For this review, take the finished solid that the model builds, in its own axes (mm). Face numbers are marked on the shaded views. A direction names the side the tool comes from. Round coordinates to 2 decimals unless told otherwise and drop trailing zeros. Write each loop counter-clockwise with the first axis right and the second up, starting at its lowest first coordinate (ties: lowest second). Pieces come first, ordered by that corner, then holes.
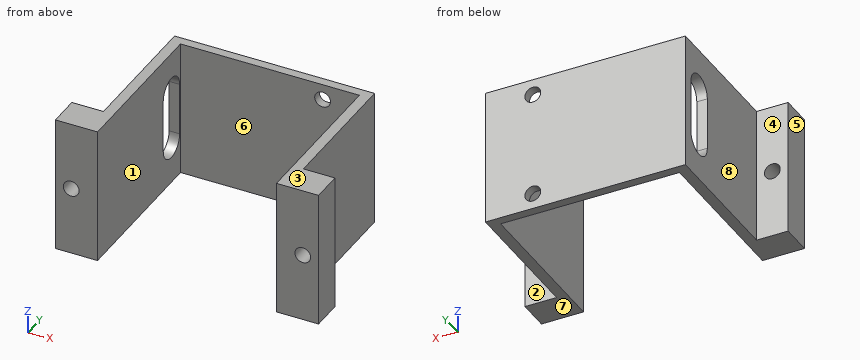
from build123d import *

# Parameters (mm, degrees)
BOSS_EXTRUDE1_DEPTH = 26
SKETCH2_R           = 1.5
CUT_EXTRUDE1_DEPTH  = 48.117375685
SKETCH3_R           = 1.5
CUT_EXTRUDE2_DEPTH  = 45.463468151
CUT_EXTRUDE3_DEPTH  = 10


with BuildPart() as part:
    # Sketch1 → Boss-Extrude1 (new body)
    with BuildSketch(Plane.XY):
        Polygon((-25, -16), (-17, -16), (-17, 14.315789474), (17, 14.315789474), (17, -16), (25, -16), (25, -10), (19, -10), (19, 16), (-19, 16), (-19, -10), (-25, -10), align=None)
    extrude(amount=BOSS_EXTRUDE1_DEPTH)

    # Sketch2 → Cut-Extrude1 (cut, through all)
    with BuildSketch(Plane.XZ.offset(-14.315789474)):
        with Locations(Location((10, 23, 0), (0, 0, 270))):
            Circle(SKETCH2_R)
        with Locations(Location((10, 3, 0), (0, 0, 270))):
            Circle(SKETCH2_R)
    extrude(amount=-CUT_EXTRUDE1_DEPTH, mode=Mode.SUBTRACT)

    # Sketch3 → Cut-Extrude2 (cut, through all)
    with BuildSketch(Plane(origin=(0, -10, 0), x_dir=(1, 0, 0), z_dir=(0, 1, 0))):
        with Locations(Location((22, -13, 0), (0, 0, 180))):
            Circle(SKETCH3_R)
        with Locations(Location((-22, -13, 0), (0, 0, 180))):
            Circle(SKETCH3_R)
    extrude(amount=-CUT_EXTRUDE2_DEPTH, mode=Mode.SUBTRACT)

    # Sketch4 → Cut-Extrude3 (cut)
    with BuildSketch(Plane.ZY.offset(19)):
        with BuildLine():
            Line((8, 14), (18, 14))
            ThreePointArc((18, 14), (21, 11), (18, 8))
            Line((18, 8), (8, 8))
            ThreePointArc((8, 8), (5, 11), (8, 14))
        make_face()
    extrude(amount=-CUT_EXTRUDE3_DEPTH, mode=Mode.SUBTRACT)


solid = part.part
(1) We need section A-A, the plane z = 3. Give the boundary of the cut face in (x, y).
Geometry check:
outline: (-25, -16) - (-17, -16) - (-17, 14.32) - (8.5, 14.32) - (8.5, 16) - (-19, 16) - (-19, -10) - (-25, -10) - close; (11.5, 14.32) - (17, 14.32) - (17, -16) - (25, -16) - (25, -10) - (19, -10) - (19, 16) - (11.5, 16) - close
(2) We need section D-D, the plane z = 13. Give the boundary of the cut face in (x, y).
Geometry check:
outline: (-25, -16) - (-23.5, -16) - (-23.5, -10) - (-25, -10) - close; (-20.5, -16) - (-17, -16) - (-17, 8) - (-19, 8) - (-19, -10) - (-20.5, -10) - close; (-19, 14) - (-17, 14) - (-17, 14.32) - (17, 14.32) - (17, -16) - (20.5, -16) - (20.5, -10) - (19, -10) - (19, 16) - (-19, 16) - close; (23.5, -16) - (25, -16) - (25, -10) - (23.5, -10) - close
(3) Mouldability with a two-part tool opening along X and no side actions: class the marked faces 6, 7 and 8 as pulls with the +X half, pulls with the -X half, needs draft (parallel to the pull), parting line crosses it, or undercut.
Geometry check:
face 6: undercut
face 7: needs draft
face 8: pulls with the -X half
(4) For pin 1 Ø6 at (y, z) = (-9.5, 13) entering from -X; pin 2 Ø3 at (x, z) = (13, 16) entering from -Y; pin 3 Ø5 at (x, z) = (22, 10) entering from +Y; pin 4 Ø1 at (y, z) = (-2.5, 7.5) entering from -X, all flat-tipped, find the tip position at first contact; note any pin that passes through.
Geometry check:
pin 1: stops at x = -25
pin 2: stops at y = 14.32
pin 3: stops at y = -10
pin 4: stops at x = -19
(5) We need section C-C, the plane y = 11. Give the boundary of the cut face in (x, z).
Geometry check:
outline: (-19, 0) - (-17, 0) - (-17, 5) - (-19, 5) - close; (-19, 21) - (-17, 21) - (-17, 26) - (-19, 26) - close; (17, 0) - (19, 0) - (19, 26) - (17, 26) - close
(6) For the marked faces 1, 2, 3, 4 and 5, list the 3-axis set-ups (+Z, -Z, +X, -X, +Y, -Y) from which the entire face can be reached by the end or side of a thin tool; tool diameter is ignored.
Geometry check:
face 1: +Z, -Z, -Y
face 2: +Z, -Z, +X, +Y
face 3: +Z, +X, -X, +Y, -Y
face 4: +Z, -Z, -X, +Y
face 5: +Z, -Z, -X, +Y, -Y
(7) For line 1 along X through (y, z) = (-1, 20.25); line 2 along X through (y, z) = (15.1, 3); line 3 along Z through (x, y) = (-22, -13.55), list the stretches that pass through material, from the lowest coordinate up.
Geometry check:
line 1: x = -19 to -17, 17 to 19
line 2: x = -19 to 8.5, 11.5 to 19
line 3: z = 0 to 11.5, 14.5 to 26
(8) We need section B-B, the plane x = 22. Give the boundary of the cut face in (y, z), and give its area (3 significant figures).
Geometry check:
outline: (-16, 0) - (-10, 0) - (-10, 11.5) - (-16, 11.5) - close; (-16, 14.5) - (-10, 14.5) - (-10, 26) - (-16, 26) - close
area: 138 mm2
